```python
from build123d import *

# Parameters (mm, degrees)
SKETCH1_R           = 38.1
BOSS_EXTRUDE1_DEPTH = 177.80000000000007
SKETCH3_R           = 35.559999999999995
CUT_EXTRUDE1_DEPTH  = 152.4
FILLET2_R           = 1.27
FILLET3_R           = 1.27
SKETCH9_R           = 7.62
CUT_EXTRUDE2_DEPTH  = 165.1
SKETCH8_W           = 162.58314194957535
SKETCH8_H           = 382.9318112434521
CUT_EXTRUDE3_DEPTH  = 76.2
BOSS_EXTRUDE2_DEPTH = 7.619999999999988
SKETCH14_R          = 1.5239999999999987
CUT_EXTRUDE4_DEPTH  = 22.859999999999992
FILLET5_R           = 2.539999999999999
BOSS_EXTRUDE3_DEPTH = 7.619999999999988
FILLET6_R           = 2.539999999999999
SKETCH16_R          = 1.524000000000002
CUT_EXTRUDE5_DEPTH  = 22.859999999999992


with BuildPart() as part:
    # Sketch1 → Boss-Extrude1 (new body)
    with BuildSketch(Plane.XY):
        with Locations(Location((0, 0, 0), (0, 0, 180))):
            Circle(SKETCH1_R)
    extrude(amount=BOSS_EXTRUDE1_DEPTH)

    # Sketch2 → Revolve1 (revolve)
    with BuildSketch(Plane.XY.offset(177.80000000000007)):
        with BuildLine():
            Line((0, 38.1), (0, -38.1))
            ThreePointArc((0, -38.1), (-38.1, 4.67e-15), (0, 38.1))
        make_face()
    revolve(axis=Axis((0, 38.1, 177.80000000000007), (0, -1, 0)))

    # Sketch3 → Cut-Extrude1 (cut)
    with BuildSketch(Plane(origin=(0, 0, 12.7), x_dir=(-1, 0, 0), z_dir=(0, 0, -1))):
        Circle(SKETCH3_R)
    extrude(amount=-CUT_EXTRUDE1_DEPTH, mode=Mode.SUBTRACT)

    # Sketch6 → Revolve2 (revolve)
    with BuildSketch(Plane(origin=(0, 0, 0), x_dir=(-1, 0, 0), z_dir=(0, -1, 0))):
        with BuildLine():
            Line((0, -22.265951698074105), (0, 130.1340483019259))
            Line((0, 130.1340483019259), (-25.4, 130.1340483019259))
            add(Edge.make_bspline(
                [(-25.4, -22.265951698074105), (-27.209474215272646, -11.435886390625324), (-47.26531015507889, 9.698536893320565), (-32.8781656152221, 32.20916869017141), (-21.12597121495262, 47.868344338725585), (-46.9742504639721, 77.09905148430619), (-20.88415964856982, 111.24461293700098), (-25.4, 130.1340483019259)],
                knots=[0, 0, 0, 0, 0.261326759387534, 0.3596065034464086, 0.4835247043674423, 0.5659559263177129, 1, 1, 1, 1], degree=3))
            Line((-25.4, -22.265951698074105), (0, -22.265951698074105))
        make_face()
    revolve(axis=Axis((0, 0, 22.265951698074105), (0, 0, -1)))

    # Fillet2
    fillet2_edges = [part.edges().sort_by_distance(p)[0] for p in [
        (38.1, -9.33e-15, 0),
    ]]
    fillet(fillet2_edges, radius=FILLET2_R)

    # Fillet3
    fillet3_edges = [part.edges().sort_by_distance(p)[0] for p in [
        (-25.4, -3.11e-15, -130.1340483019259),
    ]]
    fillet(fillet3_edges, radius=FILLET3_R)

    # Sketch9 → Cut-Extrude2 (cut)
    with BuildSketch(Plane(origin=(0, 0, -130.1340483019259), x_dir=(-1, 0, 0), z_dir=(0, 0, -1))):
        Circle(SKETCH9_R)
    extrude(amount=-CUT_EXTRUDE2_DEPTH, mode=Mode.SUBTRACT)

    # Sketch8 → Cut-Extrude3 (cut)
    with BuildSketch(Plane(origin=(0, 0, 0), x_dir=(-1, 0, 0), z_dir=(0, -1, 0))):
        with Locations((4.054997145320982, -34.07619336508105)):
            Rectangle(SKETCH8_W, SKETCH8_H)
    extrude(amount=-CUT_EXTRUDE3_DEPTH, mode=Mode.SUBTRACT)

    # Sketch13 → Boss-Extrude2 (add)
    with BuildSketch(Plane(origin=(-35.559999999999995, 0, 0), x_dir=(0, 0, -1), z_dir=(1, 0, 0))):
        Polygon((-88.89999999999999, -10.159999999999995), (-99.06, -10.159999999999997), (-99.06, -20.319999999999997), (-78.74, -20.319999999999997), (-78.74, -10.159999999999995), align=None)
    extrude(amount=BOSS_EXTRUDE2_DEPTH)

    # Sketch14 → Cut-Extrude4 (cut)
    with BuildSketch(Plane(origin=(0, 0, 78.74), x_dir=(-1, 0, 0), z_dir=(0, 0, -1))):
        with Locations((29.94604004289414, -14.16356154450682)):
            Circle(SKETCH14_R)
    extrude(amount=-CUT_EXTRUDE4_DEPTH, mode=Mode.SUBTRACT)

    # Fillet5
    fillet5_edges = [part.edges().sort_by_distance(p)[0] for p in [
        (-35.559999999999995, -20.319999999999997, 88.9),
    ]]
    fillet(fillet5_edges, radius=FILLET5_R)

    # Sketch15 → Boss-Extrude3 (add)
    with BuildSketch(Plane.ZY.offset(-35.55999999999999)):
        Polygon((88.89999999999999, -10.159999999999995), (78.74, -10.159999999999997), (78.74, -20.319999999999997), (99.06, -20.319999999999997), (99.06, -10.159999999999995), align=None)
    extrude(amount=BOSS_EXTRUDE3_DEPTH)

    # Fillet6
    fillet6_edges = [part.edges().sort_by_distance(p)[0] for p in [
        (35.55999999999999, -20.319999999999997, 88.9),
    ]]
    fillet(fillet6_edges, radius=FILLET6_R)

    # Sketch16 → Cut-Extrude5 (cut)
    with BuildSketch(Plane(origin=(0, 0, 78.74), x_dir=(-1, 0, 0), z_dir=(0, 0, -1))):
        with Locations((-30.332583398218205, -13.54198617207203)):
            Circle(SKETCH16_R)
    extrude(amount=-CUT_EXTRUDE5_DEPTH, mode=Mode.SUBTRACT)


solid = part.part
```
Geometry: final body of the model. Coordinates: model frame, mm. A direction names the side the tool comes from. Round coordinates to 2 decimals unless told otherwise and drop trailing zeros. Loops run counter-clockwise (first coordinate to the right, second up) from the corner with the lowest first, then second, coordinate; pieces in that order, holes last. Notation, with made-up numbers: (32.5, 12.25) -> (52.5, 12.25) arc R38 cw to (52.5, 51.25) -> close; hole circle Ø3 at (-33.75, -34). An arc over 180 degrees is marked (long way). Write each question's results on one line, items separated by ' | '.
Item 1: Set-up query: faces 5 (the face through (0, -11, -130.134)), 6 (the face through (0.17, -7.62, -55)), 7 (the face through (0, -13, 22.266)), 8 (the face through (3, -30, 12.7)). Return all of +Z, -Z, +X, -X, +Y, -Y with unobstructed straight access to the full face (end or side cutting, diameter ignored); none if empty.
Answers below:
face 5: -Z, +X, -X, +Y, -Y | face 6: -Z, +Y | face 7: +Y | face 8: none
Item 2: Pin query (flat end, axial travel): pin 1 Ø3.5 at (x, y) = (-29.95, -14.16) entering from +Z; pin 2 Ø5 at (x, y) = (-16.5, -24) entering from +Z; pin 3 Ø12 at (y, z) = (-8, 100.5) entering from +X. Return the tip coordinate at first contact, or that it passes through.
Answers below:
pin 1: stops at z = 199.41 | pin 2: stops at z = 205.05 | pin 3: stops at x = 38.05
Item 3: Line query: probe 1 along Z at (x, y) = (14, -12.5); probe 2 along Z at (x, y) = (25, -26); probe 3 along Y at (x, z) = (-21, 20.5). Output: solid intervals per line, ascending. Write a range as [from, to].
Answers below:
probe 1: z = [-130.13, 22.27], [165.1, 210.96] | probe 2: z = [-26.98, -0.42], [0, 190.07] | probe 3: y = [-31.79, -28.7], [-14.98, 0]
Item 4: Pull-direction query (X, two-part tool) for faces 1 (the face through (31, -10.16, 89)), 2 (the face through (-31.1, -12.9, 99.06)), 3 (the face through (-0.84, -38.09, 88.3)), 4 (the face through (10, 0, 16)); classes: pulls with the +X half, pulls with the -X half, needs draft (parallel to the pull), parting line crosses it, or undercut.
Answers below:
face 1: undercut | face 2: undercut | face 3: parting line crosses it | face 4: needs draft
Item 5: Cut plane A-A on z = 144.5. Return the cut outline in (x, y), and give its area (3 significant figures).
Answers below:
outline: (-38.1, 0) arc R38.1 ccw to (38.1, 0) -> (35.56, 0) arc R35.56 cw to (-35.56, 0) -> close | area: 294 mm²
